Could you check a few things on this model? Use its own coordinates, in mm. A direction names the side the tool comes from. Give positions to 0.01 mm unless a question says otherwise; leave off trailing zeros. Loops run counter-clockwise (first coordinate to the right, second up) from the corner with the lowest first, then second, coordinate; pieces in that order, holes last. Notation, with made-up numbers: M 49.5,67 L 81.5,67 A16 ccw 81.5,93 Z; hole C -23.5,85 d5. An arc over 180 degrees is marked long. Return JSON: item names as keys, results as strings. Group by question number.
1. If we section it at B-B (z = -3): Write out the boundary of the cut face in (x, y), plus the area to 3 significant figures.
2. If we section it at A-A (x = 4): Write out the boundary of the cut face in (y, z), plus the area to 3 significant figures.
3. If we section it at D-D (z = 0.75): Write out the boundary of the cut face in (x, y).
4. If we section it at C-C (y = 8): Write out the boundary of the cut face in (x, z).
5. For faces 1 (the flat face through (0, 13, -4.08)), 2 (the flat face through (0.82, 13.26, -4.83)), 3 (the flat face through (-0.82, 13.26, -4.83)), 4 (the flat face through (0.38, -7.24, 0.89)), which set-ups out of +Z, -Z, +X, -X, +Y, -Y let a thin tool reach every point of the face, with its end or its side?
6. Please list where these lines run through material, in increasing order: line 1 (Z direction, x = -25, y = -5.5); line 2 (Z direction, x = 9.5, y = 13); line 3 (Y direction, x = -8, z = -0.25).
7. If we mould it in two halves opening along Z, with no side actions, what happens to faces 5 (the flat face through (0.38, -7.29, 0)), 6 (the flat face through (0, 12.331, -5)), 7 (the flat face through (0, 13.531, -3))? For each: +Z half, -Z half, draft (parallel to the pull), parting line (faces both ways), or undercut.
8. For pin 1 (5 mm diameter, centred on x = 1.5, y = 9, fed in from +Z); pin 2 (1.4 mm diameter, centred on x = -0.5, z = -3, fed in from -Y); pin 3 (5 mm diameter, centred on x = -20.5, y = -4, fed in from +Z), each with a flat end and sliding along its axis, tell me the tip position at first contact or that it passes through.
```python
from build123d import *

# Parameters (mm, degrees)
EXTRUDE_1_DEPTH      = 27
SKETCH_2_W           = 9
SKETCH_2_H           = 4
CUT_EXTRUDE_1_DEPTH  = 4
SKETCH_3_W           = 9
SKETCH_3_H           = 3.038101075
EXTRUDE_2_DEPTH      = 3
SKETCH_4_R           = 1.5
CUT_EXTRUDE_2_DEPTH  = 9
EXTRUDE_3_DEPTH      = 2
CUT_EXTRUDE_8_DEPTH  = 3.887469
SKETCH_8_W           = 8.610608055
SKETCH_8_H           = 13.248031464
CUT_EXTRUDE_9_DEPTH  = 54
EXTRUDE_4_DEPTH      = 54
SKETCH_12_W          = 24
SKETCH_12_H          = 6.005920689
SKETCH_12_H_2        = 6.032486627
EXTRUDE_6_DEPTH      = 2.215161
EXTRUDE_7_DEPTH      = 54
CUT_EXTRUDE_11_DEPTH = 54


with BuildPart() as part:
    # 草图1 → 凸台-拉伸1 (new body, symmetric)
    with BuildSketch(Plane(origin=(0, 0, 0), x_dir=(0, 0, -1), z_dir=(1, 0, 0))):
        Polygon((6.496390194, -5.234874936), (6.496390194, -1.191259859), (6.496390194, 1.388117725), (6.496390194, 3.400940667), (2.492073736, 5.926640843), (1.992780388, 6.907616744), (1.992780388, 8.966437233), (1.992780388, 13.434908234), (1.992780388, 15.531060696), (0, 15.531060696), (0, 13.265125064), (0, 9.02431695), (0, 5.531060696), (1.075983727, 5.531060696), (2.127060271, 3.7449116), (2.127060271, 3.316049082), (3.852001832, 3.316049082), (3.852001832, -5.234874936), align=None)
    extrude(amount=EXTRUDE_1_DEPTH, both=True)

    # 草图2 → 切除-拉伸1 (cut)
    with BuildSketch(Plane(origin=(0, 0, -6.496390194), x_dir=(-1, 0, 0), z_dir=(0, 0, -1))):
        with Locations((0, -3.734874936)):
            Rectangle(SKETCH_2_W, SKETCH_2_H)
    extrude(amount=-CUT_EXTRUDE_1_DEPTH, mode=Mode.SUBTRACT)

    # 草图3 → 凸台-拉伸2 (add)
    with BuildSketch(Plane(origin=(0, 0, -6.496390194), x_dir=(-1, 0, 0), z_dir=(0, 0, -1))):
        with Locations((0, -0.215824399)):
            Rectangle(SKETCH_3_W, SKETCH_3_H)
    extrude(amount=EXTRUDE_2_DEPTH)

    # 草图4 → 切除-拉伸2 (cut)
    with BuildSketch(Plane.XZ.offset(1.734874936)):
        with Locations((0, -6.102001832)):
            Circle(SKETCH_4_R)
    extrude(amount=-CUT_EXTRUDE_2_DEPTH, mode=Mode.SUBTRACT)

    # 草图6 → 凸台-拉伸3 (add, symmetric)
    with BuildSketch(Plane(origin=(0, 0, 0), x_dir=(0, 0, -1), z_dir=(1, 0, 0))):
        Polygon((1.880249614, 15.531060696), (5.880249614, 15.531060696), (5.880249614, 12.331060696), (4.080249614, 12.331060696), (4.080249614, 13.531060696), (2.0593477, 13.531060696), (1.880249614, 13.531060696), align=None)
    extrude(amount=EXTRUDE_3_DEPTH, both=True)

    # 草图7 → 切除-拉伸8 (cut)
    with BuildSketch(Plane(origin=(0, 0, -5.880249614), x_dir=(-1, 0, 0), z_dir=(0, 0, -1))):
        with BuildLine():
            Line((1, 13.831060696), (0.52341558, 12.331060696))
            Line((0.52341558, 12.331060696), (2, 12.331060696))
            Line((2, 12.331060696), (2, 15.531060696))
            Line((2, 15.531060696), (1.723060875, 14.659423543))
            ThreePointArc((1.723060875, 14.659423543), (1.447645575, 14.170073989), (1, 13.831060696))
        make_face()
        with BuildLine():
            ThreePointArc((-1.723060875, 14.659423543), (-1.447645575, 14.170073989), (-1, 13.831060696))
            Line((-1, 13.831060696), (-0.52341558, 12.331060696))
            Line((-0.52341558, 12.331060696), (-2, 12.331060696))
            Line((-2, 12.331060696), (-2, 15.531060696))
            Line((-2, 15.531060696), (-1.723060875, 14.659423543))
        make_face()
    extrude(amount=-CUT_EXTRUDE_8_DEPTH, mode=Mode.SUBTRACT)

    # 草图8 → 切除-拉伸9 (cut)
    with BuildSketch(Plane.ZY.offset(27)):
        with Locations((-8.09764747, -1.373941145)):
            Rectangle(SKETCH_8_W, SKETCH_8_H)
    extrude(amount=-CUT_EXTRUDE_9_DEPTH, mode=Mode.SUBTRACT)

    # 草图9 → 凸台-拉伸4 (add)
    with BuildSketch(Plane.ZY.offset(27)):
        Polygon((-2.215161152, 3.316049082), (-2.127060271, 3.316049082), (-2.215161152, 0.39188408), (-2.215161152, -5.614036609), (-3.792343442, -5.614036609), (-3.792343442, 3.316049082), align=None)
    extrude(amount=-EXTRUDE_4_DEPTH)

    # 草图12 → 凸台-拉伸6 (add)
    with BuildSketch(Plane.XY.offset(-2.215161152)):
        with Locations((-15, -2.611076265)):
            Rectangle(SKETCH_12_W, SKETCH_12_H)
        with Locations((15, -2.597793296)):
            Rectangle(SKETCH_12_W, SKETCH_12_H_2)
    extrude(amount=EXTRUDE_6_DEPTH)

    # 草图14 → 凸台-拉伸7 (add)
    with BuildSketch(Plane(origin=(27, 0, 0), x_dir=(0, 0, -1), z_dir=(1, 0, 0))):
        Polygon((0, 5.531060696), (0, 0.203028752), (0, -5.614036609), (-1.811628389, -8.919351055), (-1.370090128, -8.919351055), (1.414080713, -5.614036609), (1.992780388, 6.907616744), (0, 6.907616744), align=None)
    extrude(amount=-EXTRUDE_7_DEPTH)

    # 草图15 → 切除-拉伸11 (cut)
    with BuildSketch(Plane(origin=(27, 0, 0), x_dir=(0, 0, -1), z_dir=(1, 0, 0))):
        Polygon((1.992780388, 6.907616744), (1.414080713, -5.614036609), (3.792343442, -5.614036609), (3.792343442, 5.106503009), align=None)
    extrude(amount=-CUT_EXTRUDE_11_DEPTH, mode=Mode.SUBTRACT)


solid = part.part
```
Answer:
{
 "1": {"outline": "M -2,15.53 L -1.72,14.66 A1.38 ccw -1,13.83 L -0.9,13.53 L 0.9,13.53 L 1,13.83 A1.38 ccw 1.72,14.66 L 2,15.53 Z", "area": "6.24 mm²"},
 "2": {"outline": "M -8.92,1.37 L -5.61,-1.41 L 6.91,-1.99 L 15.53,-1.99 L 15.53,0 L -5.61,0 L -8.92,1.81 Z", "area": "41.6 mm²"},
 "3": {"outline": "M -27,-8.18 L 27,-8.18 L 27,-6.98 L -27,-6.98 Z"},
 "4": {"outline": "M -27,-1.99 L 27,-1.99 L 27,0 L -27,0 Z"},
 "5": {"face 1": "+X, -X, -Y", "face 2": "-Z, +X, -Y", "face 3": "-Z, -X, -Y", "face 4": "+Z, +X, -X, +Y"},
 "6": {"line 1": "z = -1.42 to 0", "line 2": "z = -1.99 to 0", "line 3": "y = -7 to 15.53"},
 "7": {"face 5": "-Z half", "face 6": "draft", "face 7": "undercut"},
 "8": {"pin 1": "stops at z = 0", "pin 2": "stops at y = 13.53", "pin 3": "stops at z = 0.49"}
}
